from build123d import *

# Parameters (mm, degrees)
F0_W          = 6.35
F0_H          = 4.7625
F0_W_2        = 4.5974
F0_W_3        = 1.016
F0_H_2        = 3.6544946585
F2_W          = 12.7
F2_H          = 1.5875
F3_DEPTH      = 0.79375
F3_DEPTH_BACK = 0.79375


with BuildPart() as f1:
    # F0 (on Front) → F1 (revolve)
    with BuildSketch(Plane.XZ):
        Rectangle(F0_W, F0_H)
        with Locations((5.4737, 0)):
            Rectangle(F0_W_2, F0_H)
        with Locations((-5.4737, 0)):
            Rectangle(F0_W_2, F0_H)
        Polygon((14.1224, 2.38125), (7.7724, 2.38125), (7.7724, -2.38125), (14.1224, -2.38125), (14.1224, 1.2732446585), align=None)
        with Locations((-10.9474, 0)):
            Rectangle(F0_W, F0_H)
        with Locations((-14.6304, 0)):
            Rectangle(F0_W_3, F0_H)
        with Locations((14.6304, -0.5540026708)):
            Rectangle(F0_W_3, F0_H_2)
        Polygon((-15.1384, -2.38125), (-15.1384, 2.38125), (-15.1384, 3.96875), (-34.1884, 3.96875), (-34.1884, 2.38125), (-34.1884, -0.79375), (-34.1884, -2.38125), align=None)
        Polygon((15.1384, 1.2732446585), (15.1384, -2.38125), (16.7259, -2.38125), (16.7259, 2.38125), (15.1384, 2.38125), align=None)
        Polygon((-59.5884, -2.38125), (-34.1884, -2.38125), (-34.1884, -0.79375), (-34.1884, 2.38125), (-59.5884, 2.38125), align=None)
    revolve(axis=Axis((0, 0, -2.38125), (-1, 0, 0)))

    # F2 (on Front) → F3 (cut, two sides)
    with BuildSketch(Plane.XZ) as f3_sk:
        with Locations((-53.2384, 1.6244021334)):
            Rectangle(F2_W, F2_H)
    extrude(amount=-F3_DEPTH, mode=Mode.SUBTRACT)
    extrude(f3_sk.sketch, amount=F3_DEPTH_BACK, mode=Mode.SUBTRACT)


solid = f1.part
The listing builds one solid part. Answer for the finished solid, in the listing's coordinates (mm). A direction names the side the tool comes from. Round coordinates to 2 decimals unless told otherwise and drop trailing zeros. Order: outer loops, then holes, each group sorted by start corner. A loop starts at its lowest first (then second) coordinate and runs counter-clockwise, first axis right, second up. Notation, with made-up numbers: (-20.5, 73.5) -> (-12.5, 73.5) arc R6 cw to (-12.5, 80.5) -> close; hole circle Ø1 at (-4, 71.5). An arc over 180 degrees is marked (long way). Put each result on its own line as item: value.
Q1. Section A-A, the plane y = 0 is taken. Write down the section's boundary in (x, z), and give its area (3 significant figures).
Results list:
outline: (-59.59, -7.14) -> (-34.19, -7.14) -> (-34.19, -8.73) -> (-15.14, -8.73) -> (-15.14, -7.14) -> (14.12, -7.14) -> (14.12, -6.04) -> (15.14, -6.04) -> (15.14, -7.14) -> (16.73, -7.14) -> (16.73, 2.38) -> (15.14, 2.38) -> (15.14, 1.27) -> (14.12, 1.27) -> (14.12, 2.38) -> (-15.14, 2.38) -> (-15.14, 3.97) -> (-34.19, 3.97) -> (-34.19, 2.38) -> (-46.89, 2.38) -> (-46.89, 0.83) -> (-59.59, 0.83) -> close
area: 765 mm^2
Q2. Section C-C, the plane z = -1.75 is taken. Write down the section's boundary in (x, y).
Results list:
outline: (-59.59, -4.72) -> (-34.19, -4.72) -> (-34.19, -6.32) -> (-15.14, -6.32) -> (-15.14, -4.72) -> (14.12, -4.72) -> (14.12, -3.6) -> (15.14, -3.6) -> (15.14, -4.72) -> (16.73, -4.72) -> (16.73, 4.72) -> (15.14, 4.72) -> (15.14, 3.6) -> (14.12, 3.6) -> (14.12, 4.72) -> (-15.14, 4.72) -> (-15.14, 6.32) -> (-34.19, 6.32) -> (-34.19, 4.72) -> (-59.59, 4.72) -> close
Q3. Section D-D, the plane y = 3 is taken. Write down the section's boundary in (x, z), and give its area (3 significant figures).
Results list:
outline: (-59.59, -6.08) -> (-34.19, -6.08) -> (-34.19, -7.98) -> (-15.14, -7.98) -> (-15.14, -6.08) -> (14.12, -6.08) -> (14.12, -4.47) -> (15.14, -4.47) -> (15.14, -6.08) -> (16.73, -6.08) -> (16.73, 1.32) -> (15.14, 1.32) -> (15.14, -0.29) -> (14.12, -0.29) -> (14.12, 1.32) -> (-15.14, 1.32) -> (-15.14, 3.22) -> (-34.19, 3.22) -> (-34.19, 1.32) -> (-59.59, 1.32) -> close
area: 634 mm^2
Q4. Each of these flat-tipped pins is pushed along its axis until it touches: P1, Ø5, axis at x = 0.5, z = -4.5, coming from the +Y side; P2, Ø5, axis at y = 4, z = 2.5, coming from the +X side; P3, Ø4, axis at x = -12.5, y = -0.5, coming from the +Z side; P4, Ø1.5, axis at x = -1.5, y = 4, coming from the +Z side. Where does it stop, or does it pass through?
Results list:
P1: y = 4.76
P2: x = 16.73
P3: z = 2.38
P4: z = 1.1
Q5. Consider line 1 along X through (y, z) = (-1, 1.5); line 2 along X through (y, z) = (4, 2); line 3 along Z through (x, y) = (-56, 0). Determine where each line is inside the solid, lowest interval first.
Results list:
line 1: -59.59 to 14.12, 15.14 to 16.73
line 2: -34.19 to -15.14
line 3: -7.14 to 0.83
Q6. Which of the six approach directions +Z, -Z, +X, -X, +Y, -Y give full straight-line access (tool end or side, diameter ignored) to faces 1 (the cylindrical face through (-0.71, -4.65, -3.41)), 2 (the cylindrical face through (14.6, -2.2, -5.3)), 3 (the flat face through (-46.888, 0, 2)), 4 (the flat face through (-34.188, 5, -1))?
Results list:
face 1: +X
face 2: none
face 3: +Z, -X
face 4: -X
Q7. Section B-B, the plane x = -31 is taken. Write down the section's boundary in (y, z).
Results list:
outline: circle Ø12.7 at (0, -2.38)
Q8. Determine the mould class of faces 5 (the flat face through (-59.588, 0, -2)), 6 (the cylindrical face through (-24.797, -2.432, 3.485)), 7 (the flat face through (-53, -0.794, 2)) for opening direction Y: pulls with the +Y half, pulls with the -Y half, needs draft (parallel to the pull), parting line crosses it, or undercut.
Results list:
face 5: needs draft
face 6: parting line crosses it
face 7: undercut
